Could you check a few things on this model? Use its own coordinates, in mm. Round coordinates to 2 decimals unless told otherwise and drop trailing zeros. Loops run counter-clockwise (first coordinate to the right, second up) from the corner with the lowest first, then second, coordinate; pieces in that order, holes last. Notation, with made-up numbers: (28.25, 18.5) -> (36.25, 18.5) arc R19 cw to (36.25, 36.5) -> close; hole circle Ø4 at (53.5, 67). An arc over 180 degrees is marked (long way). Put each result on its own line as item: value. Start each with the question number.
1. I need wall thicknesses on line 1 (X direction, y = -1.85, z = 21); line 2 (Z direction, x = -26, y = -1.85); line 3 (Z direction, x = 29, y = -1.7). Which ranges of each line are inside material? Lowest first, please. Write a range as [from, to].
2. Imagine slicing it at C-C, the plane x = 26. Please give me the cut outline in (y, z), and give its area (3 significant figures).
3. I'm going to push flat-ended pins straight in: P1, Ø10, axis at x = 22, z = 15.5, coming from the +Y side; P2, Ø5.5, axis at x = 26, z = 21, coming from the +Y side. Where does each tip first touch, or does it pass through?
4. Imagine slicing it at B-B, the plane y = -2.8. Please give me the cut outline in (x, z), and give its area (3 significant figures).
5. Imagine slicing it at A-A, the plane z = 21. Please give me the cut outline in (x, y).
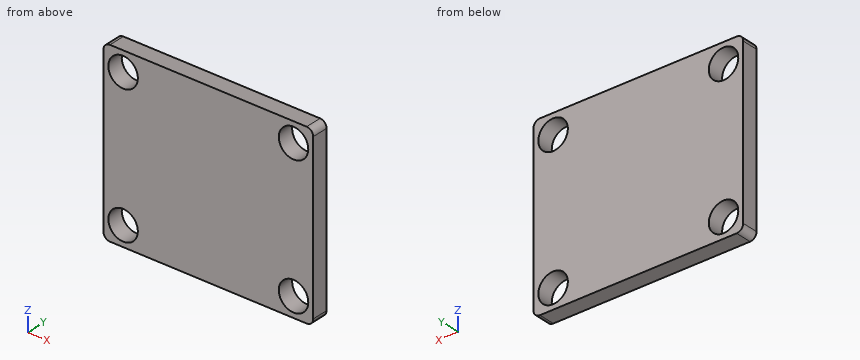
Autodesk Inventor part; units mm, degrees
ref_plane "YZ Plane" through (0, 0, 0) normal (1, 0, 0) x (0, 1, 0)
ref_plane "XZ Plane" through (0, 0, 0) normal (0, 1, 0) x (-1, 0, 0)
ref_plane "XY Plane" through (0, 0, 0) normal (0, 0, 1) x (1, 0, 0)
sketch "Sketch1" plane through (0, 0, 0) normal (0, 1, 0) x (-1, 0, 0)
  line L0 (32, 27) -> (-32, 27)
  line L1 (-32, 27) -> (-32, -27)
  line L2 (-32, -27) -> (32, -27)
  line L3 (32, -27) -> (32, 27)
  point P0 (0, -27)
  point P1 (32, 0)
  point P2 (0, 0)
  dimension "d13" = 64
  dimension "d14" = 54
extrude "Extrusion1" add sketch "Sketch1" against normal blind 5
fillet "Fillet1" radius 2 4 edges at (-32, -2.5, 27) (-32, -2.5, -27) (32, -2.5, 27) (32, -2.5, -27)
sketch "Sketch2" plane through (0, -5, 0) normal (0, -1, 0) x (1, 0, 0)
  arc A0 (30, -27) -> (32, -25) centre (30, -25) ccw
  line L0 (32, -25) -> (32, 25)
  arc A1 (32, 25) -> (30, 27) centre (30, 25) ccw
  line L1 (30, 27) -> (-30, 27)
  arc A2 (-30, 27) -> (-32, 25) centre (-30, 25) ccw
  line L2 (-32, 25) -> (-32, -25)
  arc A3 (-32, -25) -> (-30, -27) centre (-30, -25) ccw
  line L3 (-30, -27) -> (30, -27)
  line L4 (20, 15) -> (-20, 15) construction
  line L5 (-20, 15) -> (-20, -15) construction
  line L6 (-20, -15) -> (20, -15) construction
  line L7 (20, -15) -> (20, 15) construction
  line L8 (-32, 27) -> (32, 27) construction
  line L9 (32, 27) -> (32, -27) construction
  line L10 (32, -27) -> (-32, -27) construction
  line L11 (-32, -27) -> (-32, 27) construction
  line L12 (-32, 27) -> (-20, 15) construction
  line L13 (-32, -27) -> (-20, -15) construction
  line L14 (32, -27) -> (20, -15) construction
  line L15 (32, 27) -> (20, 15) construction
  point P0 (0, 0)
  point P1 (0, 0)
  point P2 (0, -15)
  point P3 (20, 0)
  point P4 (0, 27)
  point P5 (32, 0)
  point P6 (-32, 0)
  point P7 (0, -27)
  point P8 (-26, -21)
  point P9 (26, -21)
  point P10 (26, 21)
  point P11 (-26, 21)
  dimension "d15" = 40
  dimension "d16" = 30
  dimension "d19" = 12
  dimension "d20" = 12
  dimension "d21" = 64
  dimension "d22" = 54
  dimension "d23" = 6
hole "Hole1" at (-26, -5, -21) at (26, -5, -21) at (26, -5, 21) at (-26, -5, 21) direction (0, 1, 0) diameter 9 end through all
properties part number "cubierta1" material "Polycarbonate, Smoke"
Entries:
1. line 1: [-32, -30.5], [-21.5, 21.5], [30.5, 32]
1. line 2: [-27, -25.5], [-16.5, 16.5], [25.5, 27]
1. line 3: [-27, -24.35], [-17.65, 17.65], [24.35, 27]
2. outline: (-5, -27) -> (0, -27) -> (0, -25.5) -> (-5, -25.5) -> close; (-5, -16.5) -> (0, -16.5) -> (0, 16.5) -> (-5, 16.5) -> close; (-5, 25.5) -> (0, 25.5) -> (0, 27) -> (-5, 27) -> close
2. area: 180 mm^2
3. P1: y = 0
3. P2: through
4. outline: (-32, -25) arc R2 ccw to (-30, -27) -> (30, -27) arc R2 ccw to (32, -25) -> (32, 25) arc R2 ccw to (30, 27) -> (-30, 27) arc R2 ccw to (-32, 25) -> close; hole circle Ø9 at (-26, -21); hole circle Ø9 at (-26, 21); hole circle Ø9 at (26, -21); hole circle Ø9 at (26, 21)
4. area: 3,200 mm^2
5. outline: (-32, -5) -> (-30.5, -5) -> (-30.5, 0) -> (-32, 0) -> close; (-21.5, -5) -> (21.5, -5) -> (21.5, 0) -> (-21.5, 0) -> close; (30.5, -5) -> (32, -5) -> (32, 0) -> (30.5, 0) -> close
